Can you work these out from the model? Positions are in its coordinate system, mm. Coordinates: 2 decimals unless noted, no trailing zeros. Loops run counter-clockwise (first coordinate to the right, second up) from the corner with the lowest first, then second, coordinate; pieces in that order, holes last. Notation, with made-up numbers: (-37.5, 19.5) -> (-13.5, 19.5) arc R11 cw to (-13.5, 26.5) -> close; hole circle Ø11 at (36, -32.75). An arc over 180 degrees is marked (long way). Put each result on its own line as item: value. Start each with the question number.
Item 1: If we section it at A-A on x = 14.9: Please give me the cut outline in (y, z).
Item 2: Will these pins go through, and if not, where does the flat tip stop? P1, Ø0.9, axis at x = -44, z = 2, coming from the -Y side; P2, Ø1.5, axis at x = -17, z = 2.5, coming from the +Y side; P3, Ø1, axis at x = -9.5, z = 2.5, coming from the -Y side; P4, Ø3, axis at x = -15.4, y = 17.2, coming from the -Z side.
Item 3: If we section it at B-B on y = 1.1: Please give me the cut outline in (x, z).
Item 4: If we section it at D-D on x = -11: Please give me the cut outline in (y, z).
Item 5: Please list where these lines run through material, in increasing order: L1, parallel to Y at x = 14.9, z = 1.45; L2, parallel to Y at x = -15.4, z = 2.3; L3, parallel to Y at x = 39.5, z = 0.1. Write a range as from..to.
Item 6: If we section it at C-C on z = 0.7: State how many separate pieces and enclosed holes the cut face has, plus the area to 3 significant figures.
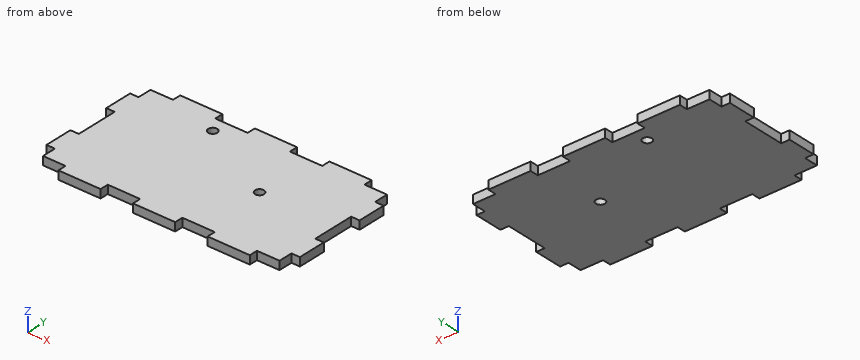
```python
from build123d import *

# Parameters (mm, degrees)
EXTRUDE_1_DEPTH     = 3
SKETCH_3_R          = 1.6
CUT_EXTRUDE_1_DEPTH = 52.809748118


with BuildPart() as part:
    # 草图1 → 凸台-拉伸1 (new body)
    with BuildSketch(Plane.XY):
        Polygon((-42, -22.5), (-34, -22.5), (-34, -25.5), (-19, -25.5), (-19, -22.5), (-7.5, -22.5), (-7.5, -25.5), (7.5, -25.5), (7.5, -22.5), (19, -22.5), (19, -25.5), (34, -25.5), (34, -22.5), (42, -22.5), (42, -17.5), (45, -17.5), (45, -7.5), (42, -7.5), (42, 7.5), (45, 7.5), (45, 17.5), (42, 17.5), (42, 22.5), (34, 22.5), (34, 25.5), (19, 25.5), (19, 22.5), (7.5, 22.5), (7.5, 25.5), (-7.5, 25.5), (-7.5, 22.5), (-19, 22.5), (-19, 25.5), (-34, 25.5), (-34, 22.5), (-42, 22.5), (-42, 17.5), (-45, 17.5), (-45, 7.5), (-42, 7.5), (-42, -7.5), (-45, -7.5), (-45, -17.5), (-42, -17.5), align=None)
    extrude(amount=EXTRUDE_1_DEPTH)

    # 草图3 → 切除-拉伸1 (cut, through all)
    with BuildSketch(Plane.XY.offset(3)):
        with Locations((-15.4, 17.2)):
            Circle(SKETCH_3_R)
        with Locations((14.9, 1.1)):
            Circle(SKETCH_3_R)
    extrude(amount=-CUT_EXTRUDE_1_DEPTH, mode=Mode.SUBTRACT)


solid = part.part
```
Solutions:
1. outline: (-22.5, 0) -> (-0.5, 0) -> (-0.5, 3) -> (-22.5, 3) -> close; (2.7, 0) -> (22.5, 0) -> (22.5, 3) -> (2.7, 3) -> close
2. P1: y = -17.5
2. P2: y = 22.5
2. P3: y = -22.5
2. P4: through
3. outline: (-42, 0) -> (13.3, 0) -> (13.3, 3) -> (-42, 3) -> close; (16.5, 0) -> (42, 0) -> (42, 3) -> (16.5, 3) -> close
4. outline: (-22.5, 0) -> (22.5, 0) -> (22.5, 3) -> (-22.5, 3) -> close
5. L1: -22.5..-0.5, 2.7..22.5
5. L2: -22.5..15.6, 18.8..22.5
5. L3: -22.5..22.5
6. separate pieces: 1
6. enclosed holes: 2
6. area: 4,150 mm^2
